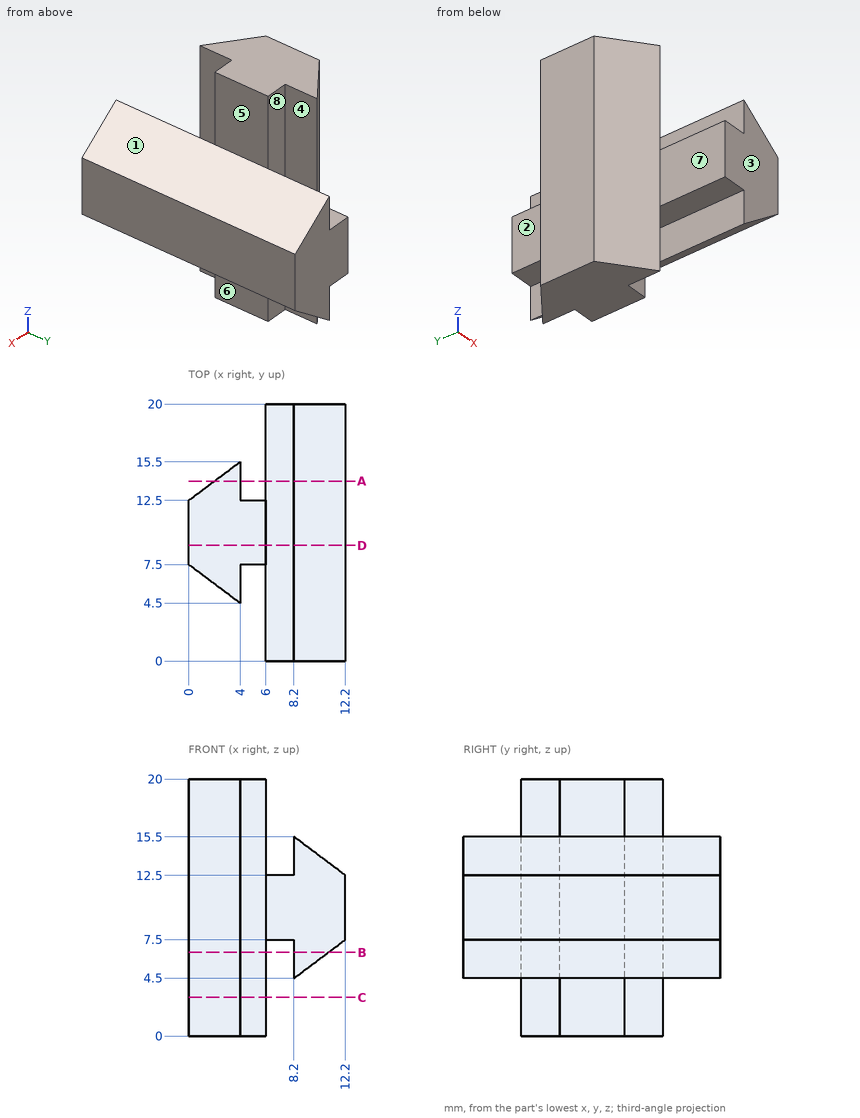
Here's the drawing with two shaded views (mm, measured from the low corner). I have some questions. A direction names the side the tool comes from. Round coordinates to 2 decimals unless told otherwise and drop trailing zeros. Loops run counter-clockwise (first coordinate to the right, second up) from the corner with the lowest first, then second, coordinate; pieces in that order, holes last.
Item 1: Suppose I cut it at B-B, the plane z = 6.5. Write out the boundary of the cut face in (x, y), then the cut area to 3 significant figures.
Item 2: If we mould it in two halves opening along X, with no side actions, what happens to the marked faces 1, 2, 3 and 4? For each: +X half, -X half, draft (parallel to the pull), parting line (faces both ways), or undercut.
Item 3: Suppose I cut it at D-D, the plane y = 9. Write out the boundary of the cut face in (x, z).
Item 4: Suppose I cut it at A-A, the plane y = 14. Write out the boundary of the cut face in (x, z).
Item 5: Suppose I cut it at C-C, the plane z = 3. Write out the boundary of the cut face in (x, y), then the cut area to 3 significant figures.
Item 6: Which directions (+Z, -Z, +X, -X, +Y, -Y) give clear straight access to the entire face, cutting with the end or side of a thin tool? Please do the marked faces 5, 6, 7 and 8.
Item 7: Will these pins go through, and if not, where does the flat tip stop? pin 1 Ø1.5 at (y, z) = (4, 9) entering from -X; pin 2 Ø1 at (x, z) = (5, 5.5) entering from +Y; pin 3 Ø1.5 at (x, z) = (2, 9) entering from -Y.
Item 8: Please list where these lines run through material, in increasing order: L1, parallel to Y at x = 5, z = 2; L2, parallel to X at y = 2.25, z = 9.25; L3, parallel to X at y = 9.25, z = 1.5.
Reported:
1. outline: (0, 7.5) - (4, 4.5) - (4, 7.5) - (6, 7.5) - (6, 12.5) - (4, 12.5) - (4, 15.5) - (0, 12.5) - close; (8.2, 0) - (10.87, 0) - (10.87, 20) - (8.2, 20) - close
1. area: 95.3 mm2
2. face 1: +X half
2. face 2: undercut
2. face 3: draft
2. face 4: undercut
3. outline: (0, 0) - (6, 0) - (6, 7.5) - (8.2, 7.5) - (8.2, 4.5) - (12.2, 7.5) - (12.2, 12.5) - (8.2, 15.5) - (8.2, 12.5) - (6, 12.5) - (6, 20) - (0, 20) - close
4. outline: (2, 0) - (4, 0) - (4, 20) - (2, 20) - close; (6, 7.5) - (8.2, 7.5) - (8.2, 4.5) - (12.2, 7.5) - (12.2, 12.5) - (8.2, 15.5) - (8.2, 12.5) - (6, 12.5) - close
5. outline: (0, 7.5) - (4, 4.5) - (4, 7.5) - (6, 7.5) - (6, 12.5) - (4, 12.5) - (4, 15.5) - (0, 12.5) - close
5. area: 42.0 mm2
6. face 5: +Z, +Y, -Y
6. face 6: -Z, +Y, -Y
6. face 7: +Z, -Z, -Y
6. face 8: +Z, -Z, +Y
7. pin 1: stops at x = 3.67
7. pin 2: stops at y = 12.5
7. pin 3: stops at y = 5.44
8. L1: y = 7.5 to 12.5
8. L2: x = 6 to 12.2
8. L3: x = 0 to 6
